Autodesk Inventor part; units mm, degrees
ref_plane "YZ Plane" through (0, 0, 0) normal (1, 0, 0) x (0, 1, 0)
ref_plane "XZ Plane" through (0, 0, 0) normal (0, 1, 0) x (-1, 0, 0)
ref_plane "XY Plane" through (0, 0, 0) normal (0, 0, 1) x (1, 0, 0)
sketch "Náčrt1" plane through (0, 0, 0) normal (0, 1, 0) x (-1, 0, 0)
  line L0 (0, -68.6) -> (0, 68.6)
  line L1 (-123.9, 0) -> (123.9, 0)
  line L2 (88.5, -49) -> (-88.5, -49)
  line L3 (-88.5, -49) -> (-88.5, 49)
  line L4 (-88.5, 49) -> (88.5, 49)
  line L5 (88.5, 49) -> (88.5, -49)
  point P0 (0, 0)
  dimension "d0" = 98
  dimension "d1" = 177
extrude "Vysunutí1" add sketch "Náčrt1" along normal blind 3
sketch "Náčrt2" plane through (0, 3, 0) normal (0, 1, 0) x (1, 0, 0)
  line L0 (88.5, 49) -> (-88.5, 49)
  line L1 (-88.5, 49) -> (-88.5, -49)
  line L2 (-88.5, -49) -> (88.5, -49)
  line L3 (88.5, -49) -> (88.5, 49)
  line L4 (88.5, 49) -> (-88.5, 49)
  line L5 (-88.5, 49) -> (-88.5, -49)
  line L6 (-88.5, 49) -> (88.5, 49)
  line L7 (88.5, 49) -> (88.5, -49)
  line L8 (88.5, -49) -> (-88.5, -49)
  line L9 (-88.5, -49) -> (-88.5, 49)
  line L10 (-85.5, -39.1) -> (-85.5, 39.1)
  line L11 (-85.5, 39.1) -> (-78.6, 39.1)
  line L12 (-78.6, 39.1) -> (-78.6, 46)
  line L13 (-78.6, 46) -> (78.6, 46)
  line L14 (78.6, 46) -> (78.6, 39.1)
  line L15 (78.6, 39.1) -> (85.5, 39.1)
  line L16 (85.5, 39.1) -> (85.5, -39.1)
  line L17 (85.5, -39.1) -> (78.6, -39.1)
  line L18 (78.6, -39.1) -> (78.6, -46)
  line L19 (78.6, -46) -> (-78.6, -46)
  line L20 (-78.6, -46) -> (-78.6, -39.1)
  line L21 (-78.6, -39.1) -> (-85.5, -39.1)
  point P0 (0, 0)
  dimension "d4" = 3
  dimension "d5" = 3
  dimension "d6" = 3
  dimension "d7" = 3
  dimension "d8" = 9.9
  dimension "d9" = 9.9
  dimension "d10" = 9.9
  dimension "d11" = 9.9
  dimension "d12" = 9.9
  dimension "d13" = 9.9
  dimension "d14" = 9.9
  dimension "d15" = 9.9
extrude "Vysunutí2" add sketch "Náčrt2" along normal blind 100
fillet "Zaoblení1" radius 3 8 edges at (-78.6, 53, -39.1) (78.6, 53, -39.1) (-78.6, 53, 39.1) (78.6, 53, 39.1) (88.5, 51.5, -49) (-88.5, 51.5, -49) (-88.5, 51.5, 49) (88.5, 51.5, 49)
sketch "Náčrt3" plane through (0, 103, 0) normal (0, 1, 0) x (1, 0, 0)
  line L0 (-88.5, 49) -> (-88.5, -49)
  line L1 (85.5, 49) -> (-85.5, 49)
  line L2 (-88.5, 46) -> (-88.5, -46)
  line L3 (-85.5, -49) -> (85.5, -49)
  line L4 (88.5, -46) -> (88.5, 46)
  arc A0 (81.6, -39.1) -> (78.6, -42.1) centre (81.6, -42.1) ccw
  line L5 (78.6, -42.1) -> (78.6, -46)
  line L6 (78.6, -46) -> (-78.6, -46)
  line L7 (-78.6, -46) -> (-78.6, -42.1)
  arc A1 (-78.6, -42.1) -> (-81.6, -39.1) centre (-81.6, -42.1) ccw
  line L8 (-81.6, -39.1) -> (-85.5, -39.1)
  line L9 (-85.5, -39.1) -> (-85.5, 39.1)
  line L10 (-85.5, 39.1) -> (-81.6, 39.1)
  arc A2 (-81.6, 39.1) -> (-78.6, 42.1) centre (-81.6, 42.1) ccw
  line L11 (-78.6, 42.1) -> (-78.6, 46)
  line L12 (-78.6, 46) -> (78.6, 46)
  line L13 (78.6, 46) -> (78.6, 42.1)
  arc A3 (78.6, 42.1) -> (81.6, 39.1) centre (81.6, 42.1) ccw
  line L14 (81.6, 39.1) -> (85.5, 39.1)
  line L15 (85.5, 39.1) -> (85.5, -39.1)
  line L16 (85.5, -39.1) -> (81.6, -39.1)
  arc A4 (85.5, -49) -> (88.5, -46) centre (85.5, -46) ccw
  arc A5 (88.5, 46) -> (85.5, 49) centre (85.5, 46) ccw
  arc A6 (-85.5, 49) -> (-88.5, 46) centre (-85.5, 46) ccw
  arc A7 (-88.5, -46) -> (-85.5, -49) centre (-85.5, -46) ccw
  point P0 (0, 0)
  point P1 (-83.55, 44.05)
  point P2 (-83.55, -44.05)
  point P3 (83.55, -44.05)
  point P4 (83.55, 44.05)
  dimension "d19" = 4.95
  dimension "d20" = 4.95
  dimension "d21" = 4.95
  dimension "d22" = 4.95
  dimension "d23" = 4.95
  dimension "d24" = 4.95
  dimension "d25" = 4.95
  dimension "d26" = 4.95
hole "Díra1" at (-83.55, 103, -44.05) at (-83.55, 103, 44.05) at (83.55, 103, 44.05) at (83.55, 103, -44.05) direction (0, -1, 0) diameter 3.9 depth 60
sketch "Náčrt4" plane through (0, 3, 0) normal (0, 1, 0) x (1, 0, 0)
  line L0 (0, 68.6) -> (0, -68.6)
  line L1 (123.9, 0) -> (-123.9, 0)
  line L2 (85.5, 39.1) -> (85.5, -39.1)
  point P0 (0, 0)
  point P1 (-18.5, 25.5)
  point P2 (77.5, 25.5)
  point P3 (-18.5, -25.5)
  point P4 (77.5, -25.5)
  dimension "d34" = 51
  dimension "d35" = 96
  dimension "d36" = 96
  dimension "d37" = 51
  dimension "d38" = 8
  dimension "d39" = 25.5
hole "Díra2" at (-18.5, 3, -25.5) at (77.5, 3, -25.5) at (-18.5, 3, 25.5) at (77.5, 3, 25.5) direction (0, -1, 0) diameter 3.4 end through all
sketch "Náčrt5" plane through (0, 3, 0) normal (0, 1, 0) x (1, 0, 0)
  line L0 (-85.5, -39.1) -> (-85.5, 39.1)
  line L1 (123.9, 0) -> (-123.9, 0)
  line L2 (-74, -38) -> (-33, -38)
  line L3 (-33, -38) -> (-33, 38)
  line L4 (-33, 38) -> (-74, 38)
  line L5 (-74, 38) -> (-74, -38)
  circle A0 centre (-18.5, 25.5) radius 1.7
  point P0 (0, 0)
  dimension "d47" = 41
  dimension "d48" = 76
  dimension "d49" = 14.5
extrude "Vysunutí3" cut sketch "Náčrt5" against normal blind 1 contours L3 L2 L5 L1 | L1 L5 L4 L3
chamfer "Zkosení1" distance 1.5 angle 45 4 edges at (77.5, 0, -27.2) (-18.5, 0, -27.2) (77.5, 0, 23.8) (-18.5, 0, 23.8)
sketch "Náčrt6" plane through (-88.5, 0, -46) normal (-1, 0, 0) x (0, 0, 1)
  line L0 (-22.6, 0) -> (114.6, 0)
  line L1 (46, 123.6) -> (46, -20.6)
  point P0 (46, 0)
  point P1 (46, 45)
  dimension "d55" = 45
hole "Díra3" at (-88.5, 45, 0) direction (1, 0, 0) diameter 15.2 depth 3
equation "\"d9\" = d8"
equation "\"d10\" = d8"
equation "\"d11\" = d8"
equation "\"d12\" = d8"
equation "\"d13\" = d8"
equation "\"d14\" = d8"
equation "\"d15\" = d8"
properties part number "box_bottom"
Build history of the part. All positions in model axes, mm. A direction names the side the tool comes from. Round coordinates to 2 decimals unless told otherwise and drop trailing zeros. Loops run counter-clockwise (first coordinate to the right, second up) from the corner with the lowest first, then second, coordinate; pieces in that order, holes last.
Item 1: Two-plate mould, pull along Z, no slides. Class faces 4 (the face through (1, 51, -49)), 5 (the face through (88.5, 51, 1)), 6 (the face through (81.617, 72.58, 43.796)): released by +Z, released by -Z, zero draft, split by the parting line, or undercut.
Item 2: Saw through at B-B (y = 18). List the corners of the cut face in (x, z).
Item 3: Saw through at C-C (x = -48). List the corners of the cut face in (y, z).
Item 4: Saw through at A-A (z = 0). List the corners of the cut face in (x, y), then the cut area to 3 significant figures.
Item 5: Pin check, flat tip, straight feed: P1, Ø6, axis at x = 7, z = 6.5, coming from the +Y side. Stop position of the tip, or through.
Item 6: Which spindle directions (+Z, -Z, +X, -X, +Y, -Y) get a long thin tool onto all of the face, cutting with end or side? Do faces 1 (the face through (-86.98, 51.74, 3.51)), 2 (the face through (78.6, 52, 44)), 3 (the face through (1, 0, 1)). Say none if no direction does.
Item 7: Drill centre lines: line 1 along X through (y, z) = (2.75, -25.5); line 2 along X through (y, z) = (89.5, 44.05); line 3 along Z through (x, y) = (-18.5, 1.8). Where is each one in solid material? Low to high.
Item 8: Saw through at D-D (z = 44.05). List the corners of the cut face in (x, y).
Worked answers:
1. face 4: released by -Z
1. face 5: zero draft
1. face 6: undercut
2. outline: (-88.5, -46) arc R3 ccw to (-85.5, -49) - (85.5, -49) arc R3 ccw to (88.5, -46) - (88.5, 46) arc R3 ccw to (85.5, 49) - (-85.5, 49) arc R3 ccw to (-88.5, 46) - close; hole (-85.5, -39.1) - (-81.6, -39.1) arc R3 cw to (-78.6, -42.1) - (-78.6, -46) - (78.6, -46) - (78.6, -42.1) arc R3 cw to (81.6, -39.1) - (85.5, -39.1) - (85.5, 39.1) - (81.6, 39.1) arc R3 cw to (78.6, 42.1) - (78.6, 46) - (-78.6, 46) - (-78.6, 42.1) arc R3 cw to (-81.6, 39.1) - (-85.5, 39.1) - close
3. outline: (0, -49) - (103, -49) - (103, -46) - (3, -46) - (3, -38) - (2, -38) - (2, 38) - (3, 38) - (3, 46) - (103, 46) - (103, 49) - (0, 49) - close
4. outline: (-88.5, 0) - (88.5, 0) - (88.5, 103) - (85.5, 103) - (85.5, 3) - (-33, 3) - (-33, 2) - (-74, 2) - (-74, 3) - (-85.5, 3) - (-85.5, 37.4) - (-88.5, 37.4) - close; (-88.5, 52.6) - (-85.5, 52.6) - (-85.5, 103) - (-88.5, 103) - close
4. area: 1,040 mm2
5. P1: stops at y = 3
6. face 1: -X
6. face 2: +Y
6. face 3: +Z, -Z, +X, -X, -Y
7. line 1: x = -88.5 to -74, -33 to -20.2, -16.8 to 75.8, 79.2 to 88.5
7. line 2: x = -88.5 to -85.5, -81.6 to -78.6, 78.6 to 81.6, 85.5 to 88.5
7. line 3: z = -49 to -27.2, -23.8 to 23.8, 27.2 to 49
8. outline: (-88.5, 0) - (88.5, 0) - (88.5, 103) - (85.5, 103) - (85.5, 43) - (81.6, 43) - (81.6, 103) - (78.6, 103) - (78.6, 3) - (-78.6, 3) - (-78.6, 103) - (-81.6, 103) - (-81.6, 43) - (-85.5, 43) - (-85.5, 103) - (-88.5, 103) - close
